Part print with two shaded views. Sizes in mm from the minimum x, y, z corner. A direction names the side the tool comes from. Round coordinates to 2 decimals unless told otherwise and drop trailing zeros. Order: outer loops, then holes, each group sorted by start corner. A loop starts at its lowest first (then second) coordinate and runs counter-clockwise, first axis right, second up. Notation, with made-up numbers: (57.5, 89) - (68.5, 89) arc R10 cw to (68.5, 93) - close; hole circle Ø2 at (-0.5, 30.25). An arc over 180 degrees is marked (long way). Write item = value, one per line.
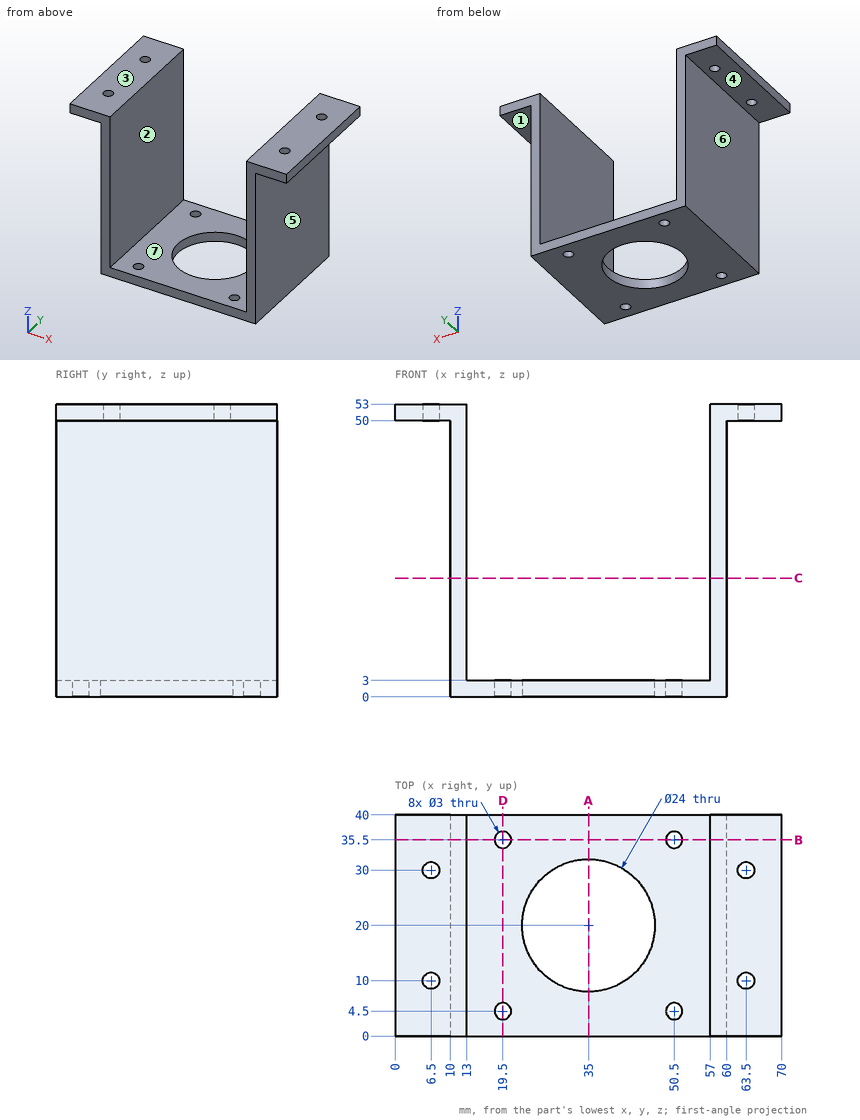
1) Cut at D-D (x = 19.5). Write the cut outline in (y, z).
Conclusion:
outline = (0, 0) - (3, 0) - (3, 3) - (0, 3) - close; (6, 0) - (34, 0) - (34, 3) - (6, 3) - close; (37, 0) - (40, 0) - (40, 3) - (37, 3) - close
2) 3-axis set-ups, long thin cutter, end or side, ignore diameter. For the marked faces 1, 2 and 3: which of +Z, -Z, +X, -X, +Y, -Y reach the whole face in a straight line?
Conclusion:
face_1 = -Z, +X, +Y, -Y
face_2 = +Z, +Y, -Y
face_3 = +Z, +X, -X, +Y, -Y
3) Mould opens along X. For the marked faces 4, 5, 6 and 7 say: +X half, -X half, draft (parallel to the pull), parting line (faces both ways), or undercut.
Conclusion:
face_4 = draft
face_5 = +X half
face_6 = -X half
face_7 = undercut
4) Cut at B-B (y = 35.5). Write the cut outline in (x, z), and give its area (3 significant figures).
Conclusion:
outline = (0, 50) - (10, 50) - (10, 0) - (18, 0) - (18, 3) - (13, 3) - (13, 53) - (0, 53) - close; (21, 0) - (49, 0) - (49, 3) - (21, 3) - close; (52, 0) - (60, 0) - (60, 50) - (70, 50) - (70, 53) - (57, 53) - (57, 3) - (52, 3) - close
area = 492 mm^2
5) Wall check: line 1 along Y through (x, z) = (6.5, 50.6); line 2 along X through (y, z) = (4.5, 1.55); line 3 along X through (y, z) = (18, 5.5). Give the ranges that are in metal, low to high.
Conclusion:
line_1 = 0 to 8.5, 11.5 to 28.5, 31.5 to 40
line_2 = 10 to 18, 21 to 49, 52 to 60
line_3 = 10 to 13, 57 to 60
6) Flat gauge pins, fed straight in: pin 1 Ø8 at (y, z) = (15.5, 5.5) entering from +X; pin 2 Ø8 at (x, y) = (4.5, 24) entering from -Z; pin 3 Ø5 at (x, y) = (63.5, 10) entering from +Z; pin 4 Ø12 at (y, z) = (21, 18) entering from -X. Where does each tip first touch, or does it go through?
Conclusion:
pin_1 = 60
pin_2 = 50
pin_3 = 53
pin_4 = 10
7) Cut at C-C (z = 21.5). Write the cut outline in (x, y), and give its area (3 significant figures).
Conclusion:
outline = (10, 0) - (13, 0) - (13, 40) - (10, 40) - close; (57, 0) - (60, 0) - (60, 40) - (57, 40) - close
area = 240 mm^2
8) Cut at A-A (x = 35). Write the cut outline in (y, z).
Conclusion:
outline = (0, 0) - (8, 0) - (8, 3) - (0, 3) - close; (32, 0) - (40, 0) - (40, 3) - (32, 3) - close
